Source: three-view drawing plus pictorial views. Frame: mm from the lowest corner of the part. A direction names the side the tool comes from. Give positions to 0.01 mm unless a question says otherwise; leave off trailing zeros. Write each loop counter-clockwise with the first axis right and the second up, starting at its lowest first coordinate (ties: lowest second). Pieces come first, ordered by that corner, then holes.
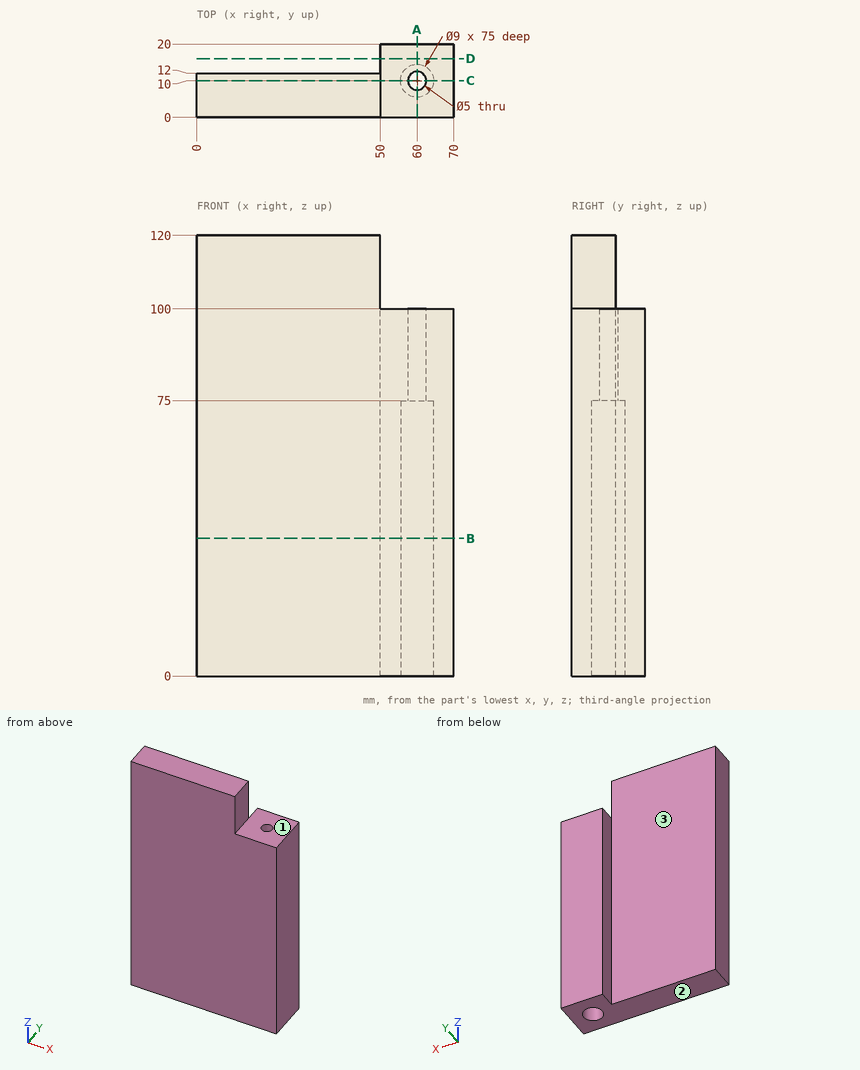
Q1. Section C-C on y = 10. Output: boundary loops of the cut face in (x, z), plus the area to 3 significant figures.
Filled sheet:
outline: (0, 0) - (55.5, 0) - (55.5, 75) - (57.5, 75) - (57.5, 100) - (50, 100) - (50, 120) - (0, 120) - close; (62.5, 75) - (64.5, 75) - (64.5, 0) - (70, 0) - (70, 100) - (62.5, 100) - close
area: 7,200 mm2
Q2. Section B-B on z = 37.5. Output: boundary loops of the cut face in (x, y), plus the area to 3 significant figures.
Filled sheet:
outline: (0, 0) - (70, 0) - (70, 20) - (50, 20) - (50, 12) - (0, 12) - close; hole circle Ø9 at (60, 10)
area: 936 mm2
Q3. Section D-D on y = 16. Output: boundary loops of the cut face in (x, z).
Filled sheet:
outline: (50, 0) - (70, 0) - (70, 100) - (50, 100) - close
Q4. Access query for the marked faces 1, 2 and 3. Directions: +Z, -Z, +X, -X, +Y, -Y. A direction counts if a zero-diameter tool reaches every point of the face in a straight line with its end or side. Return the directions, or none.
Filled sheet:
face 1: +Z, +X, +Y, -Y
face 2: -Z, +X, -X, +Y, -Y
face 3: +Z, -Z, -X, +Y
Q5. Ray query, line 1 along Y through (x, z) = (60, 93); line 2 along X through (y, z) = (13.75, 35.5); line 3 along Y through (x, z) = (59.5, 99). Return the intervals inside material, ascending.
Filled sheet:
line 1: y = 0 to 7.5, 12.5 to 20
line 2: x = 50 to 57.51, 62.49 to 70
line 3: y = 0 to 7.55, 12.45 to 20
Q6. Section A-A on x = 60. Output: boundary loops of the cut face in (y, z), plus the area to 3 significant figures.
Filled sheet:
outline: (0, 0) - (5.5, 0) - (5.5, 75) - (7.5, 75) - (7.5, 100) - (0, 100) - close; (12.5, 75) - (14.5, 75) - (14.5, 0) - (20, 0) - (20, 100) - (12.5, 100) - close
area: 1,200 mm2
Q7. Pin query (flat end, axial travel): P1, Ø5.5, axis at x = 60, y = 10, coming from the -Z side; P2, Ø10, axis at y = 6, z = 52.5, coming from the -X side; P3, Ø3, axis at x = 31.5, z = 38.5, coming from the +Y side; P4, Ø6, axis at x = 63, y = 9.5, coming from the +Z side. Return the tip coordinate at first contact, or that it passes through.
Filled sheet:
P1: stops at z = 75
P2: stops at x = 0
P3: stops at y = 12
P4: stops at z = 100
